Geometry check sheet. Reference: the model listing, model coordinates, mm. Coordinates: 2 decimals unless noted, no trailing zeros. Order: outer loops, then holes, each group sorted by start corner. A loop starts at its lowest first (then second) coordinate and runs counter-clockwise, first axis right, second up.
```python
from build123d import *

# Parameters (mm, degrees)
SKETCH1_W           = 266.7
SKETCH1_H           = 57.15
BOSS_EXTRUDE1_DEPTH = 6.35
SKETCH3_W           = 24.892
SKETCH3_H           = 8.89
BOSS_EXTRUDE2_DEPTH = 6.35
SKETCH4_W           = 13.208
SKETCH4_H           = 13.208
CUT_EXTRUDE2_DEPTH  = 139.65846972
SKETCH5_W           = 295.464136086
SKETCH5_H           = 12.7
CUT_EXTRUDE3_DEPTH  = 139.65846972
SKETCH6_W           = 266.7
SKETCH6_H           = 12.446
BOSS_EXTRUDE3_DEPTH = 6.35
SKETCH7_W           = 253.492
SKETCH7_H           = 22.86
BOSS_EXTRUDE4_DEPTH = 6.35


with BuildPart() as part:
    # Sketch1 → Boss-Extrude1 (new body)
    with BuildSketch(Plane(origin=(0, 0, 0), x_dir=(1, 0, 0), z_dir=(0, 1, 0))):
        Rectangle(SKETCH1_W, SKETCH1_H)
    extrude(amount=BOSS_EXTRUDE1_DEPTH)

    # Sketch3 → Boss-Extrude2 (add)
    with BuildSketch(Plane(origin=(0, 0, 0), x_dir=(1, 0, 0), z_dir=(0, 1, 0))):
        with Locations((-76.2, -33.02)):
            Rectangle(SKETCH3_W, SKETCH3_H)
        with Locations((-38.1, -33.02)):
            Rectangle(SKETCH3_W, SKETCH3_H)
        with Locations((0, -33.02)):
            Rectangle(SKETCH3_W, SKETCH3_H)
        with Locations((38.1, -33.02)):
            Rectangle(SKETCH3_W, SKETCH3_H)
        with Locations((76.2, -33.02)):
            Rectangle(SKETCH3_W, SKETCH3_H)
    extrude(amount=BOSS_EXTRUDE2_DEPTH)

    # Sketch4 → Cut-Extrude2 (cut, through all)
    with BuildSketch(Plane(origin=(0, 0, 0), x_dir=(1, 0, 0), z_dir=(0, 1, 0))):
        with Locations((-133.35, 22.225)):
            Rectangle(SKETCH4_W, SKETCH4_H)
        with Locations((133.35, 22.225)):
            Rectangle(SKETCH4_W, SKETCH4_H)
        with Locations((-133.35, -3.175)):
            Rectangle(SKETCH4_W, SKETCH4_H)
        with Locations((-133.35, -28.575)):
            Rectangle(SKETCH4_W, SKETCH4_H)
        with Locations((133.35, -3.175)):
            Rectangle(SKETCH4_W, SKETCH4_H)
        with Locations((133.35, -28.575)):
            Rectangle(SKETCH4_W, SKETCH4_H)
    extrude(amount=CUT_EXTRUDE2_DEPTH, mode=Mode.SUBTRACT)

    # Sketch5 → Cut-Extrude3 (cut, through all)
    with BuildSketch(Plane(origin=(0, 6.35, 0), x_dir=(1, 0, 0), z_dir=(0, 1, 0))):
        with Locations((7.963252738, 22.225)):
            Rectangle(SKETCH5_W, SKETCH5_H)
    extrude(amount=-CUT_EXTRUDE3_DEPTH, mode=Mode.SUBTRACT)

    # Sketch6 → Boss-Extrude3 (add)
    with BuildSketch(Plane(origin=(0, 6.35, 0), x_dir=(1, 0, 0), z_dir=(0, 1, 0))):
        with Locations((0, 9.652)):
            Rectangle(SKETCH6_W, SKETCH6_H)
    extrude(amount=-BOSS_EXTRUDE3_DEPTH)

    # Sketch7 → Boss-Extrude4 (add)
    with BuildSketch(Plane(origin=(0, 6.35, 0), x_dir=(1, 0, 0), z_dir=(0, 1, 0))):
        with Locations((0, 27.305)):
            Rectangle(SKETCH7_W, SKETCH7_H)
    extrude(amount=-BOSS_EXTRUDE4_DEPTH)


solid = part.part
```
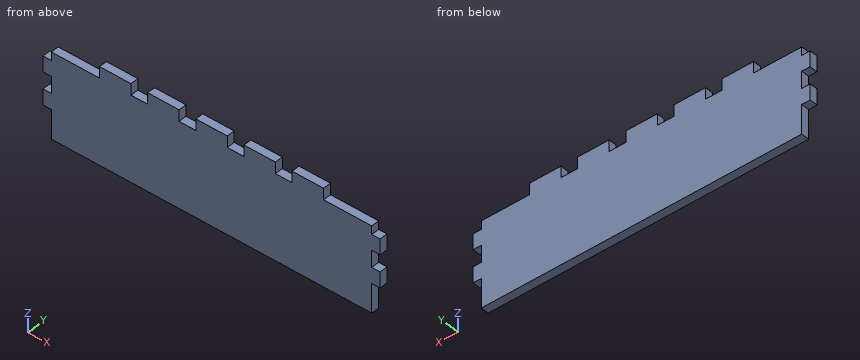
Item 1: Sectioned sample at A-A (x = 104.5). Record the cut outline in (y, z) (3 decimals), and give its area (3 significant figures).
Item 2: Thickness scan on line 1 along X through (y, z) = (3.5, 34.5); line 2 along Z through (x, y) = (-54, 1) (3 decimals); line 3 along X through (y, z) = (1.25, -25). Record the ranges inside material, lowest first.
Item 3: Depth check by flat-ended pin: P1, Ø2, axis at y = 3.5, z = -22.5, coming from the +X side; P2, Ø1.9, axis at y = 3, z = 31.5, coming from the +X side; P3, Ø3, axis at x = 113.5, y = 2.5, coming from the +Z side (3 decimals); P4, Ø12, axis at x = -84.5, z = 4.5, coming from the -Y side. Enter the tip coordinate at first touch or a pass-through.
Item 4: Sectioned sample at B-B (z = 25.5). Record the cut outline in (x, y), and give its area (3 significant figures).
Geometry check:
1. outline: (0, -38.735) - (6.35, -38.735) - (6.35, 28.575) - (0, 28.575) - close
1. area: 427 mm2
2. line 1: x = -88.65 to -63.75, -50.55 to -25.65, -12.45 to 12.45, 25.65 to 50.55, 63.75 to 88.65
2. line 2: z = -38.735 to 28.575
2. line 3: x = -126.75 to 126.75
3. P1: stops at x = 126.75
3. P2: stops at x = 88.65
3. P3: stops at z = 28.575
3. P4: stops at y = 0
4. outline: (-126.75, 0) - (126.75, 0) - (126.75, 6.35) - (-126.75, 6.35) - close
4. area: 1,610 mm2
